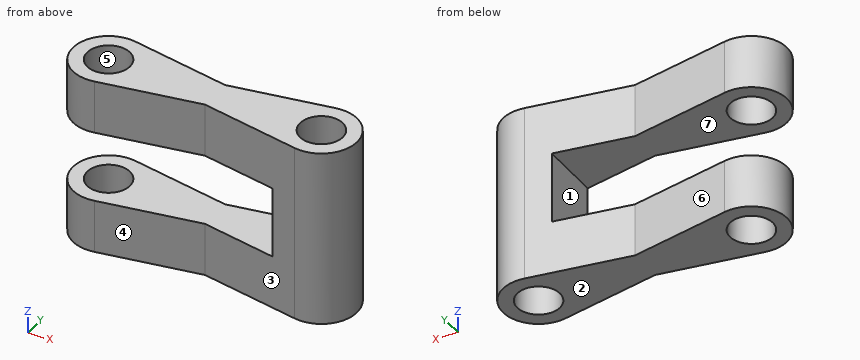
from build123d import *

# Parameters (mm, degrees)
SKETCH1_R           = 50
SKETCH1_R_2         = 30
BOSS_EXTRUDE1_DEPTH = 250
CUT_EXTRUDE1_DEPTH  = 125


with BuildPart() as part:
    # Sketch1 → Boss-Extrude1 (new body)
    with BuildSketch(Plane.XY):
        with Locations((-149.066301709, 0)):
            Circle(SKETCH1_R)
        with Locations((-149.066301709, 0)):
            Circle(SKETCH1_R_2, mode=Mode.SUBTRACT)
        with BuildLine():
            Line((0, 24.117418171), (-140.258226128, 49.218063803))
            ThreePointArc((-140.258226128, 49.218063803), (-110.72308993, 32.090467595), (-99.066301709, 0))
            ThreePointArc((-99.066301709, 0), (-110.72309003, -32.090467715), (-140.258226436, -49.218063859))
            Line((-140.258226436, -49.218063859), (0, -24.117418171))
            Line((0, -24.117418171), (140.258224826, -49.21806357))
            ThreePointArc((140.258224826, -49.21806357), (99.066301709, 3.12e-07), (140.258225441, 49.21806368))
            Line((140.258225441, 49.21806368), (0, 24.117418171))
        make_face()
        with Locations((149.066301709, 0)):
            Circle(SKETCH1_R)
        with Locations((149.066301709, 0)):
            Circle(SKETCH1_R_2, mode=Mode.SUBTRACT)
    extrude(amount=BOSS_EXTRUDE1_DEPTH)

    # Sketch2 → Cut-Extrude1 (cut, symmetric)
    with BuildSketch(Plane(origin=(0, 0, 0), x_dir=(1, 0, 0), z_dir=(0, 1, 0))):
        Polygon((-199.066301709, -75), (105.363390816, -75), (105.363390816, -125), (105.363390816, -175), (-199.066301709, -175), align=None)
    extrude(amount=CUT_EXTRUDE1_DEPTH, both=True, mode=Mode.SUBTRACT)


solid = part.part
Model file for the job. Use its own axes, mm. Face numbers are marked on the shaded views. A direction names the side the tool comes from. Give positions to 0.01 mm unless a question says otherwise; leave off trailing zeros. Loops run counter-clockwise (first coordinate to the right, second up) from the corner with the lowest first, then second, coordinate; pieces in that order, holes last. Notation, with made-up numbers: (78.5, -36.5) -> (122.5, -36.5) arc R31 ccw to (122.5, -11.5) -> close; hole circle Ø11 at (47.25, 50.5). An arc over 180 degrees is marked (long way). Use a Markdown table: item, result. Add a question column.
(1) Drop flat-ended pins along their axis: pin 1 Ø4 at (y, z) = (-38, 88.5) entering from +X (3 decimals); pin 2 Ø8 at (y, z) = (-17.5, 101.5) entering from -X; pin 3 Ø12 at (y, z) = (40, 27) entering from -X; pin 4 Ø6 at (x, y) = (144, -25) entering from +Z. Give the stop position or say it passes through.
(2) Wall check: line 1 along X through (y, z) = (-2, 14); line 2 along Z through (x, y) = (-53.5, 10.5); line 3 along X through (y, z) = (9, 16.5). Give the ranges that are in metal, low to high.
(3) Slice it at C-C on z = 63.5. List the corners of the cut face in (x, y).
(4) Slice it at B-B on x = 149.5. List the corners of the cut face in (y, z), and give its area (3 significant figures).
(5) Mould opens along Z. For the marked faces 1, 2 and 3 say: +Z half, -Z half, draft (parallel to the pull), parting line (faces both ways), or undercut.
(6) Slice it at D-D on z = 88.5. List the corners of the cut face in (x, y), and give its area (3 significant figures).
(7) Slice it at A-A on y = 0. List the corners of the cut face in (x, z).
(8) Tool access for the marked faces 4, 5, 6 and 7: list every direction of +Z, -Z, +X, -X, +Y, -Y with a clear straight run to the whole face (end or side of a thin tool).
Filled sheet:
| question | item | result |
|---|---|---|
| 1 | pin 1 | x = 183.765 |
| 1 | pin 2 | x = 105.36 |
| 1 | pin 3 | x = -185.73 |
| 1 | pin 4 | through |
| 2 | line 1 | -199.03 to -179, -119.13 to 119.13, 179 to 199.03 |
| 2 | line 2 | 0 to 75, 175 to 250 |
| 2 | line 3 | -198.25 to -177.68, -120.45 to 120.45, 177.68 to 198.25 |
| 3 | outline | (-140.26, -49.22) -> (0, -24.12) -> (140.26, -49.22) arc R50 ccw (long way) to (140.26, 49.22) -> (0, 24.12) -> (-140.26, 49.22) arc R50 ccw (long way) to start; hole circle Ø60 at (-149.07, 0); hole circle Ø60 at (149.07, 0) |
| 4 | outline | (-50, 0) -> (-30, 0) -> (-30, 250) -> (-50, 250) -> close; (30, 0) -> (50, 0) -> (50, 250) -> (30, 250) -> close |
| 4 | area | 10,000 mm2 |
| 5 | face 1 | undercut |
| 5 | face 2 | -Z half |
| 5 | face 3 | draft |
| 6 | outline | (105.36, -42.97) -> (140.26, -49.22) arc R50 ccw (long way) to (140.26, 49.22) -> (105.36, 42.97) -> close; hole circle Ø60 at (149.07, 0) |
| 6 | area | 5,190 mm2 |
| 7 | outline | (-199.07, 0) -> (-179.07, 0) -> (-179.07, 75) -> (-199.07, 75) -> close; (-199.07, 175) -> (-179.07, 175) -> (-179.07, 250) -> (-199.07, 250) -> close; (-119.07, 0) -> (119.07, 0) -> (119.07, 250) -> (-119.07, 250) -> (-119.07, 175) -> (105.36, 175) -> (105.36, 75) -> (-119.07, 75) -> close; (179.07, 0) -> (199.07, 0) -> (199.07, 250) -> (179.07, 250) -> close |
| 8 | face 4 | +Z, -Z, -Y |
| 8 | face 5 | +Z, -Z |
| 8 | face 6 | +Z, -Z, +Y |
| 8 | face 7 | -X, +Y, -Y |
